from build123d import *


with BuildPart() as part:
    # Sketch3 → Revolve1 (revolve)
    with BuildSketch(Plane.XY, mode=Mode.PRIVATE) as revolve1_sk:
        Polygon((-25, 15), (0, 15), (0, 165), (-35, 165), (-35, 155), (-25, 155), (-25, 101.665831819), (-30, 101.665831819), (-30, 15), align=None)
        Polygon((0, 165), (0, 15), (25, 15), (30, 15), (30, 101.665831819), (25, 101.665831819), (25, 155), (35, 155), (35, 165), align=None)
    revolve(revolve1_sk.sketch.rotate(Axis((0, 0, 0), (1, 0, 0)), 90), axis=Axis((0, 0, 0), (1, 0, 0)))


solid = part.part
Could you check a few things on this model? Use its own coordinates, in mm. A direction names the side the tool comes from. Give positions to 0.01 mm unless a question says otherwise; leave off trailing zeros. Order: outer loops, then holes, each group sorted by start corner. A loop starts at its lowest first (then second) coordinate and runs counter-clockwise, first axis right, second up.
1. Suppose I cut it at C-C (x = -21). Write out the boundary of the cut face in (y, z).
Answers below:
outline: circle Ø330 at (0, 0); hole circle Ø30 at (0, 0)
2. I need wall thicknesses on L1, parallel to Y at x = -28.5, z = 0; L2, parallel to Y at x = -3, z = 0; L3, parallel to X at y = 63, z = -37. Which ranges of each line are inside material? Lowest first, please.
Answers below:
L1: y = -165 to -155, -101.67 to -15, 15 to 101.67, 155 to 165
L2: y = -165 to -15, 15 to 165
L3: x = -30 to 30
3. Which directions (+Z, -Z, +X, -X, +Y, -Y) give clear straight access to the entire face, cutting with the end or side of a thin tool? Please do faces 5 (the cylindrical face through (0.42, -12.65, 8.06)), 6 (the flat face through (-25, 101, 32)), 7 (the flat face through (25, 101, -32)).
Answers below:
face 5: +X, -X
face 6: -X
face 7: +X
4. Suppose I cut it at D-D (z = 60). Write out the boundary of the cut face in (x, y), plus the area to 3 significant figures.
Answers below:
outline: (-35, -153.7) - (35, -153.7) - (35, -142.92) - (25, -142.92) - (25, -82.07) - (30, -82.07) - (30, 82.07) - (25, 82.07) - (25, 142.92) - (35, 142.92) - (35, 153.7) - (-35, 153.7) - (-35, 142.92) - (-25, 142.92) - (-25, 82.07) - (-30, 82.07) - (-30, -82.07) - (-25, -82.07) - (-25, -142.92) - (-35, -142.92) - close
area: 17,400 mm2
5. Thinking about a two-plate mould opening in Z: for faces 1 (the cylindrical face through (-29.93, 137.512, 71.523)), 2 (the cylindrical face through (-0.49, 161.076, -35.769)), 3 (the flat face through (-35, -50, -147)), 4 (the cylindrical face through (30.07, 137.512, 71.523)), which applies, +Z half, -Z half, draft (parallel to the pull), parting line (faces both ways), or undercut?
Answers below:
face 1: undercut
face 2: parting line
face 3: draft
face 4: undercut
6. For pin 1 (1.5 mm diameter, centred on y = -54, z = -20, fed in from +X); pin 2 (8 mm diameter, centred on y = -44, z = -110.5, fed in from +X); pin 3 (12 mm diameter, centred on x = -21.5, z = 24, fed in from +Y), each with a flat end and sliding along its axis, tell me the tip position at first contact or that it passes through.
Answers below:
pin 1: stops at x = 30
pin 2: stops at x = 25
pin 3: stops at y = 164.02
7. Suppose I cut it at A-A (z = 0). Write out the boundary of the cut face in (x, y).
Answers below:
outline: (-35, -165) - (35, -165) - (35, -155) - (25, -155) - (25, -101.67) - (30, -101.67) - (30, -15) - (-30, -15) - (-30, -101.67) - (-25, -101.67) - (-25, -155) - (-35, -155) - close; (-35, 155) - (-25, 155) - (-25, 101.67) - (-30, 101.67) - (-30, 15) - (30, 15) - (30, 101.67) - (25, 101.67) - (25, 155) - (35, 155) - (35, 165) - (-35, 165) - close
